Input: part model. Units: mm. Frame: model coordinates. A direction names the side the tool comes from. Coordinates: 2 decimals unless noted, no trailing zeros. Answer in a Markdown table with one row per item.
from build123d import *

# Parameters (mm, degrees)
F0_R     = 63.5
F0_R_2   = 38.1
F1_DEPTH = 127
F2_W     = 6.35
F2_H     = 40.64


with BuildPart() as f1:
    # F0 (on Front) → F1 (new body)
    with BuildSketch(Plane.XZ):
        Circle(F0_R)
        Circle(F0_R_2, mode=Mode.SUBTRACT)
    extrude(amount=F1_DEPTH)

    # F2 (on Right) → F3 (revolve, cut)
    with BuildSketch(Plane.YZ):
        with Locations((-12.907625, 63.279698)):
            Rectangle(F2_W, F2_H)
        with Locations((-22.305625, 63.279698)):
            Rectangle(F2_W, F2_H)
        with Locations((-31.703625, 63.279698)):
            Rectangle(F2_W, F2_H)
        with Locations((-41.101625, 63.279698)):
            Rectangle(F2_W, F2_H)
        with Locations((-50.499625, 63.279698)):
            Rectangle(F2_W, F2_H)
        with Locations((-59.897625, 63.279698)):
            Rectangle(F2_W, F2_H)
        with Locations((-69.295625, 63.279698)):
            Rectangle(F2_W, F2_H)
        with Locations((-78.693625, 63.279698)):
            Rectangle(F2_W, F2_H)
        with Locations((-88.091625, 63.279698)):
            Rectangle(F2_W, F2_H)
        with Locations((-97.489625, 63.279698)):
            Rectangle(F2_W, F2_H)
        with Locations((-106.887625, 63.279698)):
            Rectangle(F2_W, F2_H)
        with Locations((-116.285625, 63.279698)):
            Rectangle(F2_W, F2_H)
    revolve(axis=Axis((0, 0, 0), (0, -1, 0)), mode=Mode.SUBTRACT)

    # F4 (on Right) → F5 (revolve, cut)
    with BuildSketch(Plane.YZ):
        Polygon((-137.784824, 68.600371), (-132.080004, 38.650107), (-114.965566, 66.033214), (-90.149626, 66.033214), (-11.993693, 44.640161), (6.54695, 44.640161), (6.54695, 68.600371), align=None)
    revolve(axis=Axis((0, -127, 0), (0, -1, 0)), mode=Mode.SUBTRACT)


solid = f1.part
1) Contact query for flat-ended pins moving along their axis: pin 1 (8 mm diameter, centred on x = 24.5, y = -44.5, fed in from +Z); pin 2 (3 mm diameter, centred on x = -6.5, z = -49.5, fed in from -Y); pin 3 (4 mm diameter, centred on x = -38.5, y = -83.5, fed in from -Z). Output: stop coordinate, or through.
Resolved:
| item | result |
|---|---|
| pin 1 | stops at z = 49.83 |
| pin 2 | stops at y = -125.97 |
| pin 3 | stops at z = -51.96 |
2) Mould query, pull axis Y, two halves, no side actions, for faces 3 (the face through (-23, -9.733, 37)), 4 (the face through (-38.3, -127, 0.2)), 5 (the face through (-18.39, -72.62, 58.41)). Classes: +Y half, -Y half, draft (parallel to the pull), parting line (faces both ways), or undercut.
Resolved:
| item | result |
|---|---|
| face 3 | undercut |
| face 4 | -Y half |
| face 5 | +Y half |
3) Material intervals for probe 1 along Y at (x, z) = (32, -50.5); probe 2 along X at (y, z) = (-48, -1); probe 3 along Z at (x, y) = (0, -62), sorted ascending.
Resolved:
| item | result |
|---|---|
| probe 1 | y = -113.11 to -110.06, -103.71 to -100.66, -94.31 to -91.27, -84.92 to -81.87, -75.52 to -72.47 |
| probe 2 | x = -42.95 to -38.09, 38.09 to 42.95 |
| probe 3 | z = -42.96 to -38.1, 38.1 to 42.96 |
4) Reachability of faces 1 (the face through (13.2, -103.713, -41.4)), 2 (the face through (-13.77, -83.37, -61.99)) from +Z, -Z, +X, -X, +Y, -Y: full face, straight path, thin tool, end or side. Return the list, or none.
Resolved:
| item | result |
|---|---|
| face 1 | none |
| face 2 | +Y, -Y |
